The figure shows three views and two pictorial views of one solid part (mm, origin at its lowest corner). Answer the questions. A direction names the side the tool comes from. Round coordinates to 2 decimals unless told otherwise and drop trailing zeros. Write each loop counter-clockwise with the first axis right and the second up, starting at its lowest first coordinate (ties: lowest second). Pieces come first, ordered by that corner, then holes.
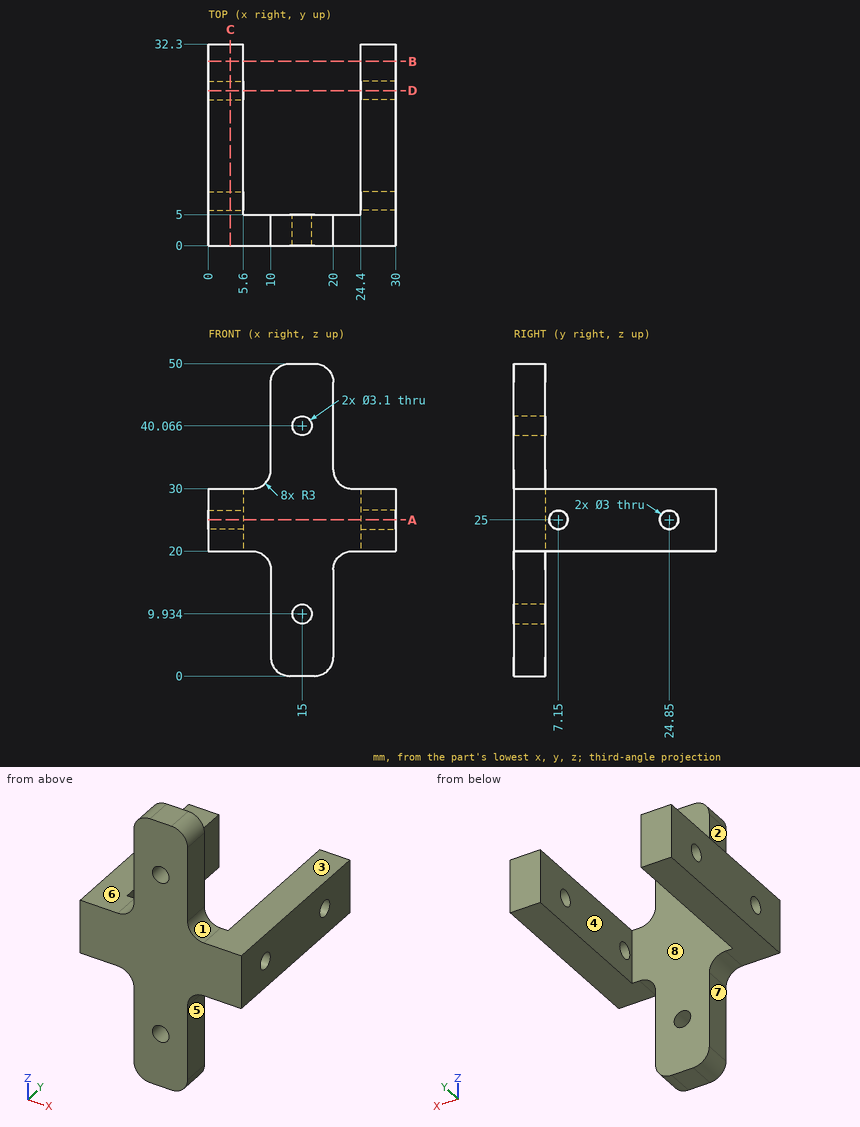
Q1. Determine the mould class of the marked faces 1, 2, 3 and 4 for opening direction X: pulls with the +X half, pulls with the -X half, needs draft (parallel to the pull), parting line crosses it, or undercut.
Verdict:
face 1: pulls with the +X half
face 2: pulls with the -X half
face 3: needs draft
face 4: undercut
Q2. Flat-ended cylindrical pins translate along their axes: pin 1 Ø2.5 at (x, z) = (15, 9.93) entering from -Y; pin 2 Ø5 at (x, z) = (15, 40.07) entering from +Y; pin 3 Ø4 at (y, z) = (1.5, 10.5) entering from +X; pin 4 Ø5.5 at (x, y) = (4, 24) entering from -Z. Find the tip coordinate at first contact, or state that the pin passes through.
Verdict:
pin 1: passes through
pin 2: stops at y = 5
pin 3: stops at x = 20
pin 4: stops at z = 20
Q3. Section C-C (x = 3.5) is taken. Determine the outline of the cut face in (y, z).
Verdict:
outline: (0, 20) - (32.3, 20) - (32.3, 30) - (0, 30) - close; hole circle Ø3 at (7.15, 25); hole circle Ø3 at (24.85, 25)
Q4. Straight lines are drawn through the part: probe 1 along Y at (x, z) = (3, 25); probe 2 along X at (y, z) = (23, 28); probe 3 along Z at (x, y) = (27.3, 24.85). For each, find the intervals that lie inside material, in ascending order.
Verdict:
probe 1: y = 0 to 5.65, 8.65 to 23.35, 26.35 to 32.3
probe 2: x = 0 to 5.6, 24.4 to 30
probe 3: z = 20 to 23.5, 26.5 to 30
Q5. Section A-A (z = 25) is taken. Determine the outline of the cut face in (x, y).
Verdict:
outline: (0, 0) - (30, 0) - (30, 5.65) - (24.4, 5.65) - (24.4, 5) - (5.6, 5) - (5.6, 5.65) - (0, 5.65) - close; (0, 8.65) - (5.6, 8.65) - (5.6, 23.35) - (0, 23.35) - close; (0, 26.35) - (5.6, 26.35) - (5.6, 32.3) - (0, 32.3) - close; (24.4, 8.65) - (30, 8.65) - (30, 23.35) - (24.4, 23.35) - close; (24.4, 26.35) - (30, 26.35) - (30, 32.3) - (24.4, 32.3) - close
Q6. Which of the six approach directions +Z, -Z, +X, -X, +Y, -Y give full straight-line access (tool end or side, diameter ignored) to the marked faces 5, 6, 7 and 8?
Verdict:
face 5: -Z, +X, +Y, -Y
face 6: +Z, -X, +Y, -Y
face 7: -Z, -X, +Y, -Y
face 8: +Z, -Z, +Y
Q7. Section B-B (y = 29.5) is taken. Determine the outline of the cut face in (x, z), then the cut area to 3 significant figures.
Verdict:
outline: (0, 20) - (5.6, 20) - (5.6, 30) - (0, 30) - close; (24.4, 20) - (30, 20) - (30, 30) - (24.4, 30) - close
area: 112 mm2
Q8. Section D-D (y = 24.85) is taken. Determine the outline of the cut face in (x, z).
Verdict:
outline: (0, 20) - (5.6, 20) - (5.6, 23.5) - (0, 23.5) - close; (0, 26.5) - (5.6, 26.5) - (5.6, 30) - (0, 30) - close; (24.4, 20) - (30, 20) - (30, 23.5) - (24.4, 23.5) - close; (24.4, 26.5) - (30, 26.5) - (30, 30) - (24.4, 30) - close
